```python
from build123d import *
from build123d.topology import SkipClean

# Parameters (mm, degrees)
SALIENTE_EXTRUIR1_REACH      = 54.713
SALIENTE_EXTRUIR1_END_RADIUS = 16
SALIENTE_EXTRUIR1_START      = -25
CROQUIS2_R                   = 7.5
CROQUIS3_W                   = 40
CROQUIS3_H                   = 40
SALIENTE_EXTRUIR2_DEPTH      = 5
REDONDEO1_R                  = 5
CROQUIS4_R                   = 1.75
CORTAR_EXTRUIR1_DEPTH        = 5


with BuildPart() as part:
    # Croquis1 → Revolución-Lámina1 (revolve)
    with BuildSketch(Plane.XY):
        with BuildLine():
            ThreePointArc((15, 0), (10.606601718, 10.606601718), (0, 15))
            Line((0, 15), (0, 16))
            ThreePointArc((0, 16), (11.313708499, 11.313708499), (16, 0))
            Line((16, 0), (15, 0))
        make_face()
    revolve(axis=Axis((0, 0, 0), (1, 0, 0)))

    # Saliente-Extruir1: up to this sphere (the profile starts outside it)
    with SkipClean():  # the faces are left unmerged after this step: merging them gives an invalid solid
        saliente_extruir1_end = Location((0, 0, 0)) * Sphere(SALIENTE_EXTRUIR1_END_RADIUS, mode=Mode.PRIVATE)
        # Croquis2 → Saliente-Extruir1 (add, up to the surface)
        with BuildSketch(Plane.ZY.offset(SALIENTE_EXTRUIR1_START), mode=Mode.PRIVATE) as saliente_extruir1_sk1:
            with Locations(Location((0, 0, 0), (0, 0, 180))):
                Circle(CROQUIS2_R)
        saliente_extruir1_tool1 = extrude(saliente_extruir1_sk1.sketch, amount=SALIENTE_EXTRUIR1_REACH, mode=Mode.PRIVATE) - saliente_extruir1_end
        add(saliente_extruir1_tool1.solids().sort_by_distance((25, 0, 0))[0])

    # Croquis3 → Saliente-Extruir2 (add)
    with BuildSketch(Plane(origin=(25, 0, 0), x_dir=(0, 0, -1), z_dir=(1, 0, 0))):
        Rectangle(CROQUIS3_W, CROQUIS3_H)
    extrude(amount=SALIENTE_EXTRUIR2_DEPTH)

    # Redondeo1
    redondeo1_edges = [part.edges().sort_by_distance(p)[0] for p in [
        (27.5, -20, -20),
        (27.5, 20, -20),
        (27.5, 20, 20),
        (27.5, -20, 20),
    ]]
    fillet(redondeo1_edges, radius=REDONDEO1_R)

    # Croquis4 → Cortar-Extruir1 (cut)
    with BuildSketch(Plane(origin=(30, 0, 0), x_dir=(0, 0, -1), z_dir=(1, 0, 0))):
        with Locations((-15.75, 15.75)):
            Circle(CROQUIS4_R)
        with Locations(Location((15.75, 15.75, 0), (0, 0, 180))):
            Circle(CROQUIS4_R)
        with Locations((15.75, -15.75)):
            Circle(CROQUIS4_R)
        with Locations(Location((-15.75, -15.75, 0), (0, 0, 180))):
            Circle(CROQUIS4_R)
    extrude(amount=-CORTAR_EXTRUIR1_DEPTH, mode=Mode.SUBTRACT)


solid = part.part
```
Here's how the part is built. I have some questions about the finished solid (model axes, mm). A direction names the side the tool comes from. Give positions to 0.01 mm unless a question says otherwise; leave off trailing zeros. Loops run counter-clockwise (first coordinate to the right, second up) from the corner with the lowest first, then second, coordinate; pieces in that order, holes last. Notation, with made-up numbers: M 17,73.5 L 52,73.5 A33 cw 52,112.5 Z; hole C -21,-39 d4. An arc over 180 degrees is marked long. Put each result on its own line as item: value. Start each with the question number.
(1) I need wall thicknesses on line 1 along Z through (x, y) = (27.5, -17); line 2 along Y through (x, z) = (26, -15.75); line 3 along X through (y, z) = (-2.5, 16.5). Which ranges of each line are inside material? Lowest first, please. Write a range as [from, to].
(2) Will these pins go through, and if not, where does the flat tip stop? pin 1 Ø2 at (x, z) = (4, 3) entering from -Y; pin 2 Ø2 at (y, z) = (13.5, -5.5) entering from -X; pin 3 Ø2 at (y, z) = (15.75, -15.75) entering from -X; pin 4 Ø8 at (x, z) = (16, 7) entering from -Y.
(3) I want a section at C-C on x = 16.75. Please give me the cut outline in (y, z).
(4) I want a section at D-D on x = 6. Please give me the cut outline in (y, z).
(5) If we mould it in two halves opening along Y, with no side actions, what happens to faces 3 (the cylindrical face through (27.535, -17.485, 15.522)), 4 (the flat face through (27, 0, -20)), 5 (the flat face through (27, 20, 0))? For each: +Y half, -Y half, draft (parallel to the pull), parting line (faces both ways), or undercut.
(6) I want a section at A-A on y = 0. Please give me the cut outline in (x, z).
(7) For faces 1 (the cylindrical face through (19.643, -6.324, -4.032)), 2 (the cylindrical face through (28, 18, 19)), which set-ups out of +Z, -Z, +X, -X, +Y, -Y let a thin tool reach every point of the face, with its end or its side?
Answer block:
1. line 1: [-19.58, -16.97], [-14.53, 14.53], [16.97, 19.58]
1. line 2: [-19.94, -17.5], [-14, 14], [17.5, 19.94]
1. line 3: [25, 30]
2. pin 1: y = -15.49
2. pin 2: x = 0
2. pin 3: through
2. pin 4: y = -8.64
3. outline: C 0,0 d15
4. outline: C 0,0 d29.66; hole C 0,0 d27.5
5. face 3: undercut
5. face 4: draft
5. face 5: +Y half
6. outline: M 0,-16 A16 ccw 14.13,-7.5 L 25,-7.5 L 25,-20 L 30,-20 L 30,20 L 25,20 L 25,7.5 L 14.13,7.5 A16 ccw 0,16 L 0,15 A15 cw 0,-15 Z
7. face 1: none
7. face 2: +Z, +X, -X, +Y
